from build123d import *

# Parameters (mm, degrees)
SKETCH_1_R        = 11
SKETCH_1_R_2      = 1.65
EXTRUDE_2_DEPTH   = 3
EXTRUDE_3_DEPTH   = 3
EXTRUDE_START     = -6
EXTRUDE_4_DEPTH   = 6
SKETCH_4_R        = 3
EXTRUDE_5_DEPTH   = 45
SKETCH_5_R        = 1.65
EXTRUDE_6_DEPTH   = 5
EXTRUDE_6_2_DEPTH = 5
SKETCH_6_R        = 3.5
EXTRUDE_7_DEPTH   = 4
EXTRUDE_7_2_DEPTH = 4


with BuildPart() as part:
    # Sketch 1 → Extrude 2 (new body)
    with BuildSketch(Plane(origin=(0, 0, 0), x_dir=(1, 0, 0), z_dir=(0, 1, 0))):
        with Locations(Location((0, 0, 0), (0, 0, 270))):
            Circle(SKETCH_1_R)
        with Locations(Location((0, -8, 0), (0, 0, 270))):
            Circle(SKETCH_1_R_2, mode=Mode.SUBTRACT)
        with Locations(Location((8, 0, 0), (0, 0, 270))):
            Circle(SKETCH_1_R_2, mode=Mode.SUBTRACT)
    extrude(amount=EXTRUDE_2_DEPTH)

    # Sketch 2 → Extrude 3 (add)
    with BuildSketch(Plane(origin=(0, 3, 0), x_dir=(1, 0, 0), z_dir=(0, 1, 0))):
        with BuildLine():
            Line((8.952279946, 6.391923323), (-5.663051219, -9.430262504))
            ThreePointArc((-5.663051219, -9.430262504), (-8.080231896, 7.463903303), (8.952279946, 6.391923323))
        make_face()
    extrude(amount=EXTRUDE_3_DEPTH)

    # Sketch 3 → Extrude 4 (add)
    with BuildSketch(Plane(origin=(0, 6, 0), x_dir=(1, 0, 0), z_dir=(0, 1, 0)).offset(EXTRUDE_START)):
        with BuildLine():
            Line((-5.663051219, -9.430262504), (8.952279946, 6.391923323))
            ThreePointArc((8.952279946, 6.391923323), (8.041723321, 7.505377141), (6.993667, 8.490501863))
            Line((6.993667, 8.490501863), (-31.406072494, 40.120550975))
            ThreePointArc((-31.406072494, 40.120550975), (-39.447295943, 39.748092317), (-39.880826602, 31.709930141))
            Line((-39.880826602, 31.709930141), (-8.543382198, -6.928969665))
            ThreePointArc((-8.543382198, -6.928969665), (-7.212475586, -8.305431712), (-5.663051219, -9.430262504))
        make_face()
    extrude(amount=EXTRUDE_4_DEPTH)

    # Sketch 4 → Extrude 5 (add)
    with BuildSketch(Plane(origin=(0, 6, 0), x_dir=(1, 0, 0), z_dir=(0, 1, 0))):
        with Locations(Location((-35.220799949, 35.48936814, 0), (0, 0, 90))):
            Circle(SKETCH_4_R)
    extrude(amount=EXTRUDE_5_DEPTH)


with BuildPart() as body_2:
    # Sketch 5 → Extrude 6 (new, symmetric)
    with BuildSketch(Plane(origin=(0, 3, 0), x_dir=(1, 0, 0), z_dir=(0, 1, 0))):
        with Locations(Location((-8, 0, 0), (0, 0, 270))):
            Circle(SKETCH_5_R)
    extrude(amount=EXTRUDE_6_DEPTH, both=True)


with BuildPart() as body_3:
    # Sketch 5 → Extrude 6 2 (new, symmetric)
    with BuildSketch(Plane(origin=(0, 3, 0), x_dir=(1, 0, 0), z_dir=(0, 1, 0))):
        with Locations(Location((0, 8, 0), (0, 0, 270))):
            Circle(SKETCH_5_R)
    extrude(amount=EXTRUDE_6_2_DEPTH, both=True)


with BuildPart() as part_1:
    add(part.part)

    # Combine 1: cut body 3, body 2
    add(body_3.part, mode=Mode.SUBTRACT)
    add(body_2.part, mode=Mode.SUBTRACT)


with BuildPart() as body_2_2:
    # Sketch 6 → Extrude 7 (new body)
    with BuildSketch(Plane(origin=(0, 3, 0), x_dir=(1, 0, 0), z_dir=(0, 1, 0))):
        with Locations(Location((0, 8, 0), (0, 0, 270))):
            Circle(SKETCH_6_R)
    extrude(amount=EXTRUDE_7_DEPTH)


with BuildPart() as body_3_2:
    # Sketch 6 → Extrude 7 2 (new body)
    with BuildSketch(Plane(origin=(0, 3, 0), x_dir=(1, 0, 0), z_dir=(0, 1, 0))):
        with Locations(Location((-8, 0, 0), (0, 0, 270))):
            Circle(SKETCH_6_R)
    extrude(amount=EXTRUDE_7_2_DEPTH)


with BuildPart() as part_2:
    add(part_1.part)

    # Combine 2: cut body 2 2, body 3 2
    add(body_2_2.part, mode=Mode.SUBTRACT)
    add(body_3_2.part, mode=Mode.SUBTRACT)


solid = part_2.part
Can you work these out from the model? Positions are in its coordinate system, mm. A direction names the side the tool comes from. Coordinates: 2 decimals unless noted, no trailing zeros. Loops run counter-clockwise (first coordinate to the right, second up) from the corner with the lowest first, then second, coordinate; pieces in that order, holes last. Notation, with made-up numbers: (25, -5) - (29, -5) arc R4 cw to (29, -1) - close; hole circle Ø7 at (-0.75, 87). An arc over 180 degrees is marked (long way). Put each result on its own line as item: value. Start each with the question number.
Item 1: Suppose I cut it at B-B (z = 0). Please give me the cut outline in (x, y), and give its area (3 significant figures).
Item 2: Suppose I cut it at D-D (z = 8). Please give me the cut outline in (x, y).
Item 3: For pin 1 (2 mm diameter, centred on x = -8, z = 0, fed in from -Y); pin 2 (5.5 mm diameter, centred on x = -8, z = 0, fed in from +Y); pin 3 (18.5 mm diameter, centred on x = 1, z = -1, fed in from +Y); pin 4 (3 mm diameter, centred on y = 36.5, z = -35, fed in from -X), each with a flat end and sliding along its axis, tell me the tip position at first contact or that it passes through.
Item 4: If I drill on line 1 along X through (y, z) = (2.4, 0); line 2 along Y through (x, z) = (-12, -19); line 3 along X through (y, z) = (3.8, 0), over which ranges is the centre line in solid material (lowest first)?
Item 5: Suppose I cut it at C-C (x = 8). Please give me the cut outline in (y, z), and give its area (3 significant figures).
Item 6: If we mould it in two halves opening along Y, with no side actions, what happens to faces 1 (the face through (1.747, 4.479, 1.408)), 2 (the face through (-15, 0, -16)), 3 (the face through (-18, 6, -18))? For each: +Y half, -Y half, draft (parallel to the pull), parting line (faces both ways), or undercut.
Item 7: Suppose I cut it at A-A (y = 5). Please give me the cut outline in (x, z), and give its area (3 significant figures).
Item 8: Which directions (+Z, -Z, +X, -X, +Y, -Y) give clear straight access to the entire face, cutting with the end or side of a thin tool? Please do faces 4 (the face through (-36.12, 28.18, -38.35)), 5 (the face through (-6.885, 1.521, -1.216)), 6 (the face through (5, 3, 4)).
Here are the results:
1. outline: (-14.16, 0) - (-9.65, 0) - (-9.65, 3) - (-11.5, 3) - (-11.5, 6) - (-14.16, 6) - close; (-6.35, 0) - (6.35, 0) - (6.35, 3) - (3.05, 3) - (3.05, 6) - (-4.5, 6) - (-4.5, 3) - (-6.35, 3) - close; (9.65, 0) - (11, 0) - (11, 3) - (9.65, 3) - close
1. area: 86.3 mm²
2. outline: (-7.55, 0) - (-1.65, 0) - (-1.65, 3) - (-4.34, 3) - (-4.34, 6) - (-7.55, 6) - close; (1.65, 0) - (7.55, 0) - (7.55, 3) - (1.65, 3) - close
3. pin 1: through
3. pin 2: y = 3
3. pin 3: y = 6
3. pin 4: x = -38.22
4. line 1: -14.16 to -9.65, -6.35 to 6.35, 9.65 to 11
4. line 2: 0 to 6
4. line 3: -14.16 to -11.5, -4.5 to 3.05
5. outline: (0, -7.55) - (6, -7.55) - (6, -5.36) - (3, -5.36) - (3, -1.65) - (0, -1.65) - close; (0, 1.65) - (3, 1.65) - (3, 7.55) - (0, 7.55) - close
5. area: 42.0 mm²
6. face 1: draft
6. face 2: -Y half
6. face 3: +Y half
7. outline: (-39.88, -31.71) arc R6 ccw to (-31.41, -40.12) - (6.99, -8.49) arc R11 ccw to (8.95, -6.39) - (-5.66, 9.43) arc R11 ccw to (-8.54, 6.93) - close; hole circle Ø7 at (-8, 0); hole circle Ø7 at (0, -8)
7. area: 883 mm²
8. face 4: +Y
8. face 5: +Y, -Y
8. face 6: +Z, +X, +Y
